Input: dimensioned drawing with shaded views. Units: mm. Origin: part minimum x, y, z. A direction names the side the tool comes from. Round coordinates to 2 decimals unless told otherwise and drop trailing zeros. Loops run counter-clockwise (first coordinate to the right, second up) from the corner with the lowest first, then second, coordinate; pieces in that order, holes last.
Item 1: Access query for the marked faces 1, 2, 3 and 4. Directions: +Z, -Z, +X, -X, +Y, -Y. A direction counts if a zero-diameter tool reaches every point of the face in a straight line with its end or side. Return the directions, or none.
Item 2: First-contact query: P1, Ø2.5, axis at x = 2, z = 3.5, coming from the +Y side; P2, Ø4, axis at x = 89.5, z = 7, coming from the -Y side; P3, Ø3, axis at y = 25.5, z = 5, coming from the +X side. Flat tips, straight axial feed; report the tip coordinate or a pass-through.
Item 3: Ray query, L1, parallel to Y at x = 79, z = 6.25; L2, parallel to X at y = 2.5, z = 2.25; L3, parallel to X at y = 16, z = 2. Return the intervals inside material, ascending.
Item 4: Section query A-A on x = 50.5. Return loops of the section in (y, z).
Item 5: Section query D-D on y = 10. Return loops of the section in (x, z).
Item 6: Section query C-C on y = 21. Return loops of the section in (x, z).
Item 7: Pull-direction query (X, two-part tool) for the marked faces 5, 6 and 7; classes: released by +X, released by -X, zero draft, split by the parting line, or undercut.
Item 8: Section query B-B on z = 1. Return loops of the section in (x, y).
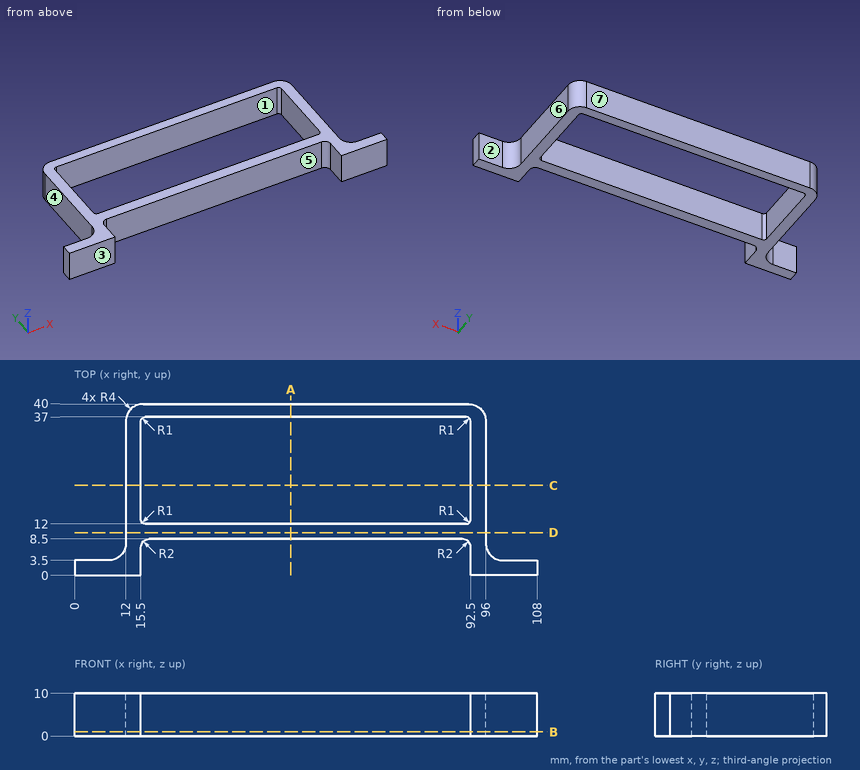
Data:
1. face 1: +Z, -Z
1. face 2: +Z, -Z, +X, +Y
1. face 3: +Z, -Z, +X, -X, -Y
1. face 4: +Z, -Z, -X, +Y
2. P1: stops at y = 3.5
2. P2: stops at y = 8.23
2. P3: stops at x = 96
3. L1: y = 8.5 to 12, 37 to 40
3. L2: x = 0 to 15.5, 92.5 to 108
3. L3: x = 12 to 15.5, 92.5 to 96
4. outline: (8.5, 0) - (12, 0) - (12, 10) - (8.5, 10) - close; (37, 0) - (40, 0) - (40, 10) - (37, 10) - close
5. outline: (12, 0) - (96, 0) - (96, 10) - (12, 10) - close
6. outline: (12, 0) - (15.5, 0) - (15.5, 10) - (12, 10) - close; (92.5, 0) - (96, 0) - (96, 10) - (92.5, 10) - close
7. face 5: undercut
7. face 6: released by +X
7. face 7: zero draft
8. outline: (0, 0) - (15.5, 0) - (15.5, 6.5) arc R2 cw to (17.5, 8.5) - (90.5, 8.5) arc R2 cw to (92.5, 6.5) - (92.5, 0) - (108, 0) - (108, 3.5) - (100, 3.5) arc R4 cw to (96, 7.5) - (96, 36) arc R4 ccw to (92, 40) - (16, 40) arc R4 ccw to (12, 36) - (12, 7.5) arc R4 cw to (8, 3.5) - (0, 3.5) - close; hole (15.5, 13) arc R1 ccw to (16.5, 12) - (91.5, 12) arc R1 ccw to (92.5, 13) - (92.5, 36) arc R1 ccw to (91.5, 37) - (16.5, 37) arc R1 ccw to (15.5, 36) - close
